Input: part model. Units: mm. Frame: model coordinates. A direction names the side the tool comes from. Coordinates: 2 decimals unless noted, no trailing zeros. Write each loop counter-clockwise with the first axis right and the second up, starting at its lowest first coordinate (ties: lowest second). Pieces come first, ordered by that corner, then holes. Notation, with made-up numbers: (-11.75, -16.5) - (-3.75, -16.5) arc R15 ccw to (-3.75, -6.5) - close; hole circle Ø2 at (-33.75, 71). An arc over 180 degrees is marked (long way). Use a Markdown table: item, result. Add a question column.
Q1. Section query C-C (x = -48). Return the cut outline in (y, z) (3 decimals).
Q2. Section query B-B (z = 7.5). Return the cut outline in (x, y), then the cut area to 3 significant figures.
Q3. Pin query (flat end, axial travel): P1, Ø5, axis at x = -21, z = 29.5, coming from the +Y side; P2, Ø17, axis at x = -12, z = 13, coming from the -Y side; P3, Ø1, axis at y = 12.5, z = 25.5, coming from the -X side; P4, Ø7, axis at y = -15.875, z = 17.78, coming from the -X side. Return the tip coordinate at first contact, or that it passes through.
Q4. Mould query, pull axis Y, two halves, no side actions, for faces 4 (the face through (-11, 18.288, 18)), 5 (the face through (-28, 1, 0)), 6 (the face through (-26, 0, 18)), 7 (the face through (-29, 6.35, 18)). Classes: released by +Y, released by -Y, zero draft, split by the parting line, or undercut.
Q5. Material intervals for probe 1 along Y at (x, z) = (-8.5, 5); probe 2 along X at (y, z) = (12, 29.5); probe 3 along X at (y, z) = (-22.5, 4), sorted ascending. Write a range as from..to.
Q6. Set-up query: faces 1 (the face through (-21.59, 13, 18)), 2 (the face through (-46.482, -20, 18)), 3 (the face through (-14, 11.938, 18)). Return all of +Z, -Z, +X, -X, +Y, -Y with unobstructed straight access to the full face (end or side cutting, diameter ignored); none if empty.
Q7. Section query D-D (y = -20.5). Return the cut outline in (x, z).
Q8. Section query A-A (z = 17.78). Return the cut outline in (x, y).
from build123d import *

# Parameters (mm, degrees)
F1_DEPTH = 35.56
F2_R     = 2.667
F3_DEPTH = 25.4
F4_R     = 5.08


with BuildPart() as f1:
    # F0 (on Top) → F1 (new body)
    with BuildSketch(Plane.XY):
        Polygon((-46.482, 0), (0, 0), (0, 18.288), (-21.59, 18.288), (-21.59, 11.938), (-6.35, 11.938), (-6.35, 6.35), (-52.832, 6.35), (-52.832, -31.75), (-46.482, -31.75), align=None)
    extrude(amount=F1_DEPTH)

    # F2 (on face) → F3 (cut)
    with BuildSketch(Plane.YZ.offset(-46.482)):
        with Locations((-15.875, 17.78)):
            Circle(F2_R)
    extrude(amount=-F3_DEPTH, mode=Mode.SUBTRACT)

    # F4
    f4_edges = [f1.edges().sort_by_distance(p)[0] for p in [
        (0, 0, 17.78),
        (0, 18.288, 17.78),
        (-21.59, 18.288, 17.78),
    ]]
    fillet(f4_edges, radius=F4_R)


solid = f1.part
Values follow:
| question | item | result |
|---|---|---|
| 1 | outline | (-31.75, 0) - (6.35, 0) - (6.35, 35.56) - (-31.75, 35.56) - close; hole circle Ø5.334 at (-15.875, 17.78) |
| 2 | outline | (-52.83, -31.75) - (-46.48, -31.75) - (-46.48, 0) - (-5.08, 0) arc R5.08 ccw to (0, 5.08) - (0, 13.21) arc R5.08 ccw to (-5.08, 18.29) - (-16.51, 18.29) arc R5.08 ccw to (-21.59, 13.21) - (-21.59, 11.94) - (-6.35, 11.94) - (-6.35, 6.35) - (-52.83, 6.35) - close |
| 2 | area | 693 mm2 |
| 3 | P1 | y = 17.88 |
| 3 | P2 | y = 0 |
| 3 | P3 | x = -21.59 |
| 3 | P4 | x = -52.83 |
| 4 | face 4 | released by +Y |
| 4 | face 5 | zero draft |
| 4 | face 6 | released by -Y |
| 4 | face 7 | undercut |
| 5 | probe 1 | 0..6.35, 11.94..18.29 |
| 5 | probe 2 | -21.59..0 |
| 5 | probe 3 | -52.83..-46.48 |
| 6 | face 1 | +Z, -Z, -X, +Y |
| 6 | face 2 | +Z, -Z, +X, -Y |
| 6 | face 3 | +Z, -Z, -X |
| 7 | outline | (-52.83, 0) - (-46.48, 0) - (-46.48, 35.56) - (-52.83, 35.56) - close |
| 8 | outline | (-52.83, -31.75) - (-46.48, -31.75) - (-46.48, -18.54) - (-52.83, -18.54) - close; (-52.83, -13.21) - (-46.48, -13.21) - (-46.48, 0) - (-5.08, 0) arc R5.08 ccw to (0, 5.08) - (0, 13.21) arc R5.08 ccw to (-5.08, 18.29) - (-16.51, 18.29) arc R5.08 ccw to (-21.59, 13.21) - (-21.59, 11.94) - (-6.35, 11.94) - (-6.35, 6.35) - (-52.83, 6.35) - close |
